from build123d import *

# Parameters (mm, degrees)
F0_W     = 141
F0_H     = 141
F0_W_2   = 136
F0_H_2   = 136
F1_DEPTH = 5
F2_DEPTH = 245
F3_R     = 22.5
F4_DEPTH = 25


with BuildPart() as f1:
    # F0 (on Top) → F1 (new body)
    with BuildSketch(Plane.XY):
        Rectangle(F0_W, F0_H)
        Rectangle(F0_W_2, F0_H_2, mode=Mode.SUBTRACT)
        Rectangle(F0_W_2, F0_H_2)
    extrude(amount=F1_DEPTH)

    # F0 (on Top) → F2 (join)
    with BuildSketch(Plane.XY):
        Rectangle(F0_W, F0_H)
        Rectangle(F0_W_2, F0_H_2, mode=Mode.SUBTRACT)
    extrude(amount=F2_DEPTH)

    # F3 (on face) → F4 (cut)
    with BuildSketch(Plane.XY.offset(5)):
        Circle(F3_R)
    extrude(amount=-F4_DEPTH, mode=Mode.SUBTRACT)


solid = f1.part
The model under review builds one solid part; all positions refer to its coordinate system, in mm. A direction names the side the tool comes from. Round coordinates to 2 decimals unless told otherwise and drop trailing zeros. Write each loop counter-clockwise with the first axis right and the second up, starting at its lowest first coordinate (ties: lowest second). Pieces come first, ordered by that corner, then holes. Notation, with made-up numbers: M 62,57 L 93,57 A28 ccw 93,81 Z; hole C -29,-32.75 d6. An arc over 180 degrees is marked long. Use a Markdown table: item, result. Add a question column.
Q1. We need section C-C, the plane z = 44.5. State the section outline as (x, y) points, plus the area to 4 significant figures.
Q2. To check wall thickness, follow line 1 (Y direction, x = -63.5, z = 160); line 2 (Y direction, x = 0, z = 1). State the ranges of each line that lie inside material, in increasing order.
Q3. We need section D-D, the plane x = -37. State the section outline as (y, z) points.
Q4. Insertion check: pin 1 (10 mm diameter, centred on x = -46, y = -8.5, fed in from -Z). The pin has a flat end and moves straight along its axis. Give the tip position at first contact, or say it passes through.
Q5. We need section A-A, the plane y = 0. State the section outline as (x, z) points, plus the area to 3 significant figures.
Q6. Machinability: for faces 4 (the face through (68, -1, 123)), 5 (the face through (-68.2, 31.7, 245)), which of the approach directions +Z, -Z, +X, -X, +Y, -Y give a long, thin tool a straight path to every point of the face, cutting with its end or side? Answer none if there is none.
Q7. The part is to be moulded in two halves that separate along X. For faces 1 (the face through (-68, -1, 123)), 2 (the face through (-17, 17, 0)), 3 (the face through (70.5, -1, 121)), say which applies: pulls with the +X half, pulls with the -X half, needs draft (parallel to the pull), parting line crosses it, or undercut.
Findings below:
| question | item | result |
|---|---|---|
| 1 | outline | M -70.5,-70.5 L 70.5,-70.5 L 70.5,70.5 L -70.5,70.5 Z; hole M -68,-68 L 68,-68 L 68,68 L -68,68 Z |
| 1 | area | 1,385 mm² |
| 2 | line 1 | y = -70.5 to -68, 68 to 70.5 |
| 2 | line 2 | y = -70.5 to -22.5, 22.5 to 70.5 |
| 3 | outline | M -70.5,0 L 70.5,0 L 70.5,245 L 68,245 L 68,5 L -68,5 L -68,245 L -70.5,245 Z |
| 4 | pin 1 | stops at z = 0 |
| 5 | outline | M -70.5,0 L -22.5,0 L -22.5,5 L -68,5 L -68,245 L -70.5,245 Z; M 22.5,0 L 70.5,0 L 70.5,245 L 68,245 L 68,5 L 22.5,5 Z |
| 5 | area | 1,680 mm² |
| 6 | face 4 | +Z |
| 6 | face 5 | +Z, +X, -X, +Y, -Y |
| 7 | face 1 | undercut |
| 7 | face 2 | needs draft |
| 7 | face 3 | pulls with the +X half |
